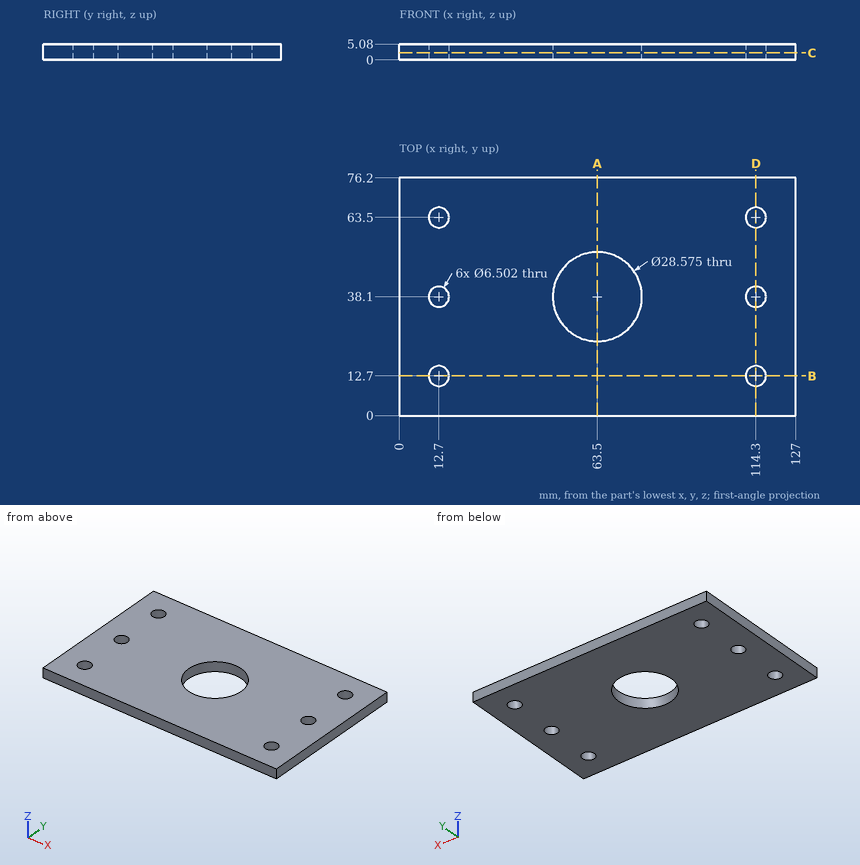
The figure shows three views and two pictorial views of one solid part (mm, origin at its lowest corner). Answer the questions. Coordinates: 2 decimals unless noted, no trailing zeros. Loops run counter-clockwise (first coordinate to the right, second up) from the corner with the lowest first, then second, coordinate; pieces in that order, holes last.
1) Find section A-A on x = 63.5. Write down the section's boundary in (y, z), then the cut area to 3 significant figures.
2) A flat-ended cylindrical pin translates along its axis: pin 1 Ø8.5 at (x, y) = (12.7, 63.5) entering from -Z. Find the tip coordinate at first contact, or state that the pin passes through.
3) Find the intervals of material crossed by L1, parallel to Y at x = 114.3, z = 1.45; L2, parallel to X at y = 13, z = 3.15; L3, parallel to Y at x = 63.5, z = 3.8, in increasing order.
4) Find section B-B on y = 12.7. Write down the section's boundary in (x, z), then the cut area to 3 significant figures.
5) Find section D-D on x = 114.3. Write down the section's boundary in (y, z).
6) Find section C-C on z = 2.2. Write down the section's boundary in (x, y) (1 decimal), then the cut area to 3 significant figures.
Values:
1. outline: (0, 0) - (23.81, 0) - (23.81, 5.08) - (0, 5.08) - close; (52.39, 0) - (76.2, 0) - (76.2, 5.08) - (52.39, 5.08) - close
1. area: 242 mm2
2. pin 1: stops at z = 0
3. L1: y = 0 to 9.45, 15.95 to 34.85, 41.35 to 60.25, 66.75 to 76.2
3. L2: x = 0 to 9.46, 15.94 to 111.06, 117.54 to 127
3. L3: y = 0 to 23.81, 52.39 to 76.2
4. outline: (0, 0) - (9.45, 0) - (9.45, 5.08) - (0, 5.08) - close; (15.95, 0) - (111.05, 0) - (111.05, 5.08) - (15.95, 5.08) - close; (117.55, 0) - (127, 0) - (127, 5.08) - (117.55, 5.08) - close
4. area: 579 mm2
5. outline: (0, 0) - (9.45, 0) - (9.45, 5.08) - (0, 5.08) - close; (15.95, 0) - (34.85, 0) - (34.85, 5.08) - (15.95, 5.08) - close; (41.35, 0) - (60.25, 0) - (60.25, 5.08) - (41.35, 5.08) - close; (66.75, 0) - (76.2, 0) - (76.2, 5.08) - (66.75, 5.08) - close
6. outline: (0, 0) - (127, 0) - (127, 76.2) - (0, 76.2) - close; hole circle Ø6.5 at (12.7, 12.7); hole circle Ø6.5 at (12.7, 38.1); hole circle Ø6.5 at (12.7, 63.5); hole circle Ø28.6 at (63.5, 38.1); hole circle Ø6.5 at (114.3, 12.7); hole circle Ø6.5 at (114.3, 38.1); hole circle Ø6.5 at (114.3, 63.5)
6. area: 8,840 mm2
